The drawing under review shows one solid part. Ordinate dimensions are in mm from its lowest x, y, z. A direction names the side the tool comes from. Give positions to 0.01 mm unless a question says otherwise; leave off trailing zeros. Order: outer loops, then holes, each group sorted by start corner. A loop starts at its lowest first (then second) coordinate and runs counter-clockwise, first axis right, second up. Notation, with made-up numbers: M 66,50.5 L 109,50.5 A30 cw 109,77.5 Z; hole C 23.5,6 d6. An arc over 180 degrees is marked long. Put each result on its own line as item: value. Start each with the question number.
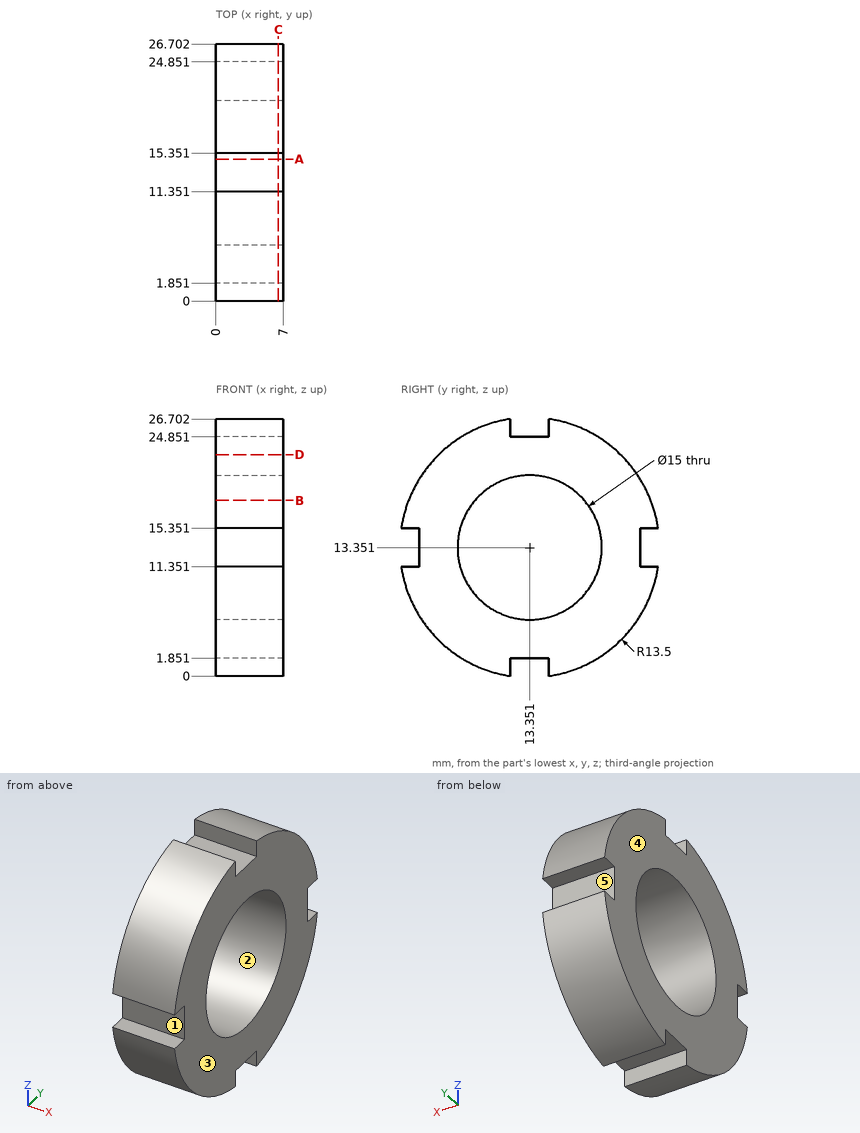
1. The part is to be moulded in two halves that separate along Y. For the marked faces 1, 2 and 3, say which applies: +Y half, -Y half, draft (parallel to the pull), parting line (faces both ways), or undercut.
2. Consider section B-B on z = 18.25. Give the boundary of the cut face in (x, y).
3. Insertion check: pin 1 (4 mm diameter, centred on x = 5.5, y = 13.5, fed in from -Z); pin 2 (2 mm diameter, centred on x = 3.5, y = 26, fed in from -Z); pin 3 (3 mm diameter, centred on x = 3, y = 8.5, fed in from +Z); pin 4 (1.5 mm diameter, centred on x = 5, y = 1.5, fed in from +Z). Each pin has a flat end and moves straight along its axis. Give the tip position at first contact, or say it passes through.
4. Consider section C-C on x = 6.5. Give the boundary of the cut face in (y, z).
5. Machinability: for the marked faces 4 and 5, which of the approach directions +Z, -Z, +X, -X, +Y, -Y give a long, thin tool a straight path to every point of the face, cutting with its end or side? Answer none if there is none.
6. Consider section D-D on z = 23. Give the boundary of the cut face in (x, y).
7. Consider section A-A on y = 14.75. Give the boundary of the cut face in (x, z).
8. To check wall thickness, follow probe 1 along Y at (x, z) = (4.75, 10.25); probe 2 along Z at (x, y) = (0.5, 11); probe 3 along Y at (x, z) = (2.25, 15). State the ranges of each line that lie inside material, in increasing order.
Returned:
1. face 1: -Y half
1. face 2: undercut
1. face 3: draft
2. outline: M 0,0.77 L 7,0.77 L 7,7.67 L 0,7.67 Z; M 0,19.03 L 7,19.03 L 7,25.93 L 0,25.93 Z
3. pin 1: stops at z = 0
3. pin 2: stops at z = 6.53
3. pin 3: stops at z = 26.43
3. pin 4: stops at z = 21.03
4. outline: M 0,11.35 A13.5 ccw 11.35,0 L 11.35,1.85 L 15.35,1.85 L 15.35,0 A13.5 ccw 26.7,11.35 L 24.85,11.35 L 24.85,15.35 L 26.7,15.35 A13.5 ccw 15.35,26.7 L 15.35,24.85 L 11.35,24.85 L 11.35,26.7 A13.5 ccw 0,15.35 L 1.85,15.35 L 1.85,11.35 Z; hole C 13.35,13.35 d15
5. face 4: +Z, -Z, -X, +Y, -Y
5. face 5: +X, -X, +Y
6. outline: M 0,3.91 L 7,3.91 L 7,22.79 L 0,22.79 Z
7. outline: M 0,1.85 L 7,1.85 L 7,5.98 L 0,5.98 Z; M 0,20.72 L 7,20.72 L 7,24.85 L 0,24.85 Z
8. probe 1: y = 0.21 to 6.52, 20.18 to 26.49
8. probe 2: z = 0.06 to 6.23, 20.47 to 26.64
8. probe 3: y = 1.85 to 6.03, 20.67 to 24.85
